Part print with two shaded views. Sizes in mm from the minimum x, y, z corner. A direction names the side the tool comes from. Coordinates: 2 decimals unless noted, no trailing zeros. Loops run counter-clockwise (first coordinate to the right, second up) from the corner with the lowest first, then second, coordinate; pieces in that order, holes last. Notation, with made-up numbers: (31, -12) -> (61, -12) arc R27 ccw to (61, 25) -> close; hole circle Ø2 at (15.25, -20.75). An arc over 180 degrees is marked (long way). Write each question's results on one line, items separated by ' | '.
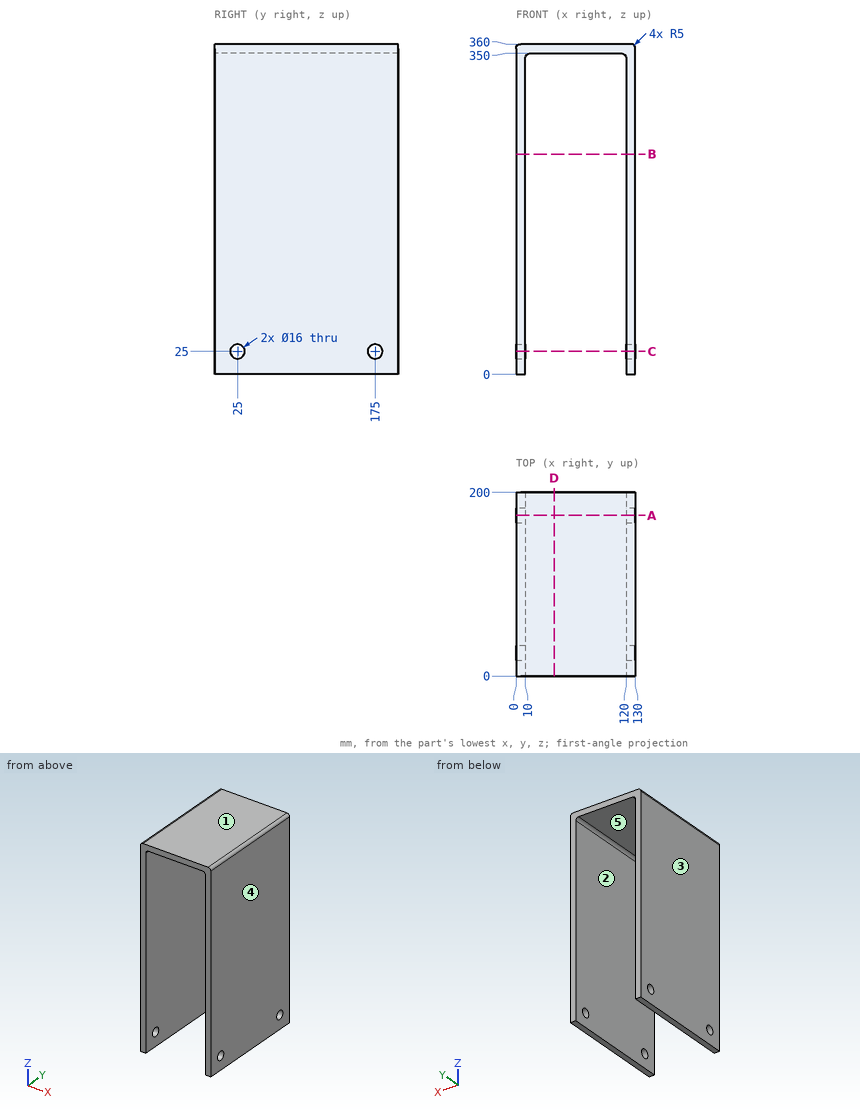
Q1. Which spindle directions (+Z, -Z, +X, -X, +Y, -Y) get a long thin tool onto all of the face, cutting with end or side? Do the marked faces 1 and 2. Say none if no direction does.
Results are:
face 1: +Z, +X, -X, +Y, -Y | face 2: -Z, +Y, -Y
Q2. Pull direction X, two halves, no side cores. Call the marked faces 3, 4 and 5: +X half, -X half, draft (parallel to the pull), parting line (faces both ways), or undercut.
Results are:
face 3: -X half | face 4: +X half | face 5: undercut
Q3. Cut at D-D on x = 41.5. Write the cut outline in (y, z), and give its area (3 significant figures).
Results are:
outline: (0, 350) -> (200, 350) -> (200, 360) -> (0, 360) -> close | area: 2,000 mm^2
Q4. Cut at A-A on y = 175. Write the cut outline in (x, z).
Results are:
outline: (0, 0) -> (10, 0) -> (10, 17) -> (0, 17) -> close; (0, 33) -> (10, 33) -> (10, 345) arc R5 cw to (15, 350) -> (115, 350) arc R5 cw to (120, 345) -> (120, 33) -> (130, 33) -> (130, 355) arc R5 ccw to (125, 360) -> (5, 360) arc R5 ccw to (0, 355) -> close; (120, 0) -> (130, 0) -> (130, 17) -> (120, 17) -> close
Q5. Cut at B-B on z = 240. Write the cut outline in (x, y), and give its area (3 significant figures).
Results are:
outline: (0, 0) -> (10, 0) -> (10, 200) -> (0, 200) -> close; (120, 0) -> (130, 0) -> (130, 200) -> (120, 200) -> close | area: 4,000 mm^2
Q6. Drop flat-ended pins along their axis: pin 1 (21 mm diameter, centred on y = 175, z = 25, fed in from -X); pin 2 (1.5 mm diameter, centred on x = 43, y = 145.5, fed in from -Z). Give the stop position or say it passes through.
Results are:
pin 1: x = 0 | pin 2: z = 350
Q7. Cut at C-C on z = 25. Write the cut outline in (x, y).
Results are:
outline: (0, 0) -> (10, 0) -> (10, 17) -> (0, 17) -> close; (0, 33) -> (10, 33) -> (10, 167) -> (0, 167) -> close; (0, 183) -> (10, 183) -> (10, 200) -> (0, 200) -> close; (120, 0) -> (130, 0) -> (130, 17) -> (120, 17) -> close; (120, 33) -> (130, 33) -> (130, 167) -> (120, 167) -> close; (120, 183) -> (130, 183) -> (130, 200) -> (120, 200) -> close
Q8. Wall check: L1, parallel to X at y = 156, z = 89; L2, parallel to Z at x = 82.5, y = 108; L3, parallel to Z at x = 124, y = 175. Give the ranges that are in metal, low to high. Write a range as from..to.
Results are:
L1: 0..10, 120..130 | L2: 350..360 | L3: 0..17, 33..360
